```python
from build123d import *

# Parameters (mm, degrees)
F0_R     = 2.9
F1_DEPTH = 15
F1_TAPER = 0.4
F2_DEPTH = 15
F2_TAPER = 0.4
F0_R_2   = 4
F3_DEPTH = 4
F4_DEPTH = 4
F5_R     = 1
F6_R     = 2.1
F7_DEPTH = 4.2
F8_DEPTH = 2.8


with BuildPart() as f1:
    # F0 (on Top) → F1 (new body)
    with BuildSketch(Plane.XY):
        Circle(F0_R)
    extrude(amount=F1_DEPTH, taper=F1_TAPER)

    # F0 (on Top) → F2 (join)
    with BuildSketch(Plane.XY):
        Circle(F0_R)
    extrude(amount=-F2_DEPTH, taper=F2_TAPER)

    # F0 (on Top) → F3 (join)
    with BuildSketch(Plane.XY):
        Circle(F0_R_2)
        Circle(F0_R, mode=Mode.SUBTRACT)
        Circle(F0_R)
    extrude(amount=F3_DEPTH)

    # F0 (on Top) → F4 (join)
    with BuildSketch(Plane.XY):
        Circle(F0_R_2)
        Circle(F0_R, mode=Mode.SUBTRACT)
        Circle(F0_R)
    extrude(amount=-F4_DEPTH)

    # F5
    f5_edges = [f1.edges().sort_by_distance(p)[0] for p in [
        (-2.795279, 0, 15),
        (-2.795279, 0, -15),
    ]]
    fillet(f5_edges, radius=F5_R)

    # F6 (on Front) → F7 (cut)
    with BuildSketch(Plane.XZ):
        Circle(F6_R)
    extrude(amount=-F7_DEPTH, mode=Mode.SUBTRACT)

    # F6 (on Front) → F8 (cut)
    with BuildSketch(Plane.XZ):
        Circle(F6_R)
    extrude(amount=F8_DEPTH, mode=Mode.SUBTRACT)


solid = f1.part
```
The model under review builds one solid part; all positions refer to its coordinate system, in mm. A direction names the side the tool comes from. Coordinates: 2 decimals unless noted, no trailing zeros. Write each loop counter-clockwise with the first axis right and the second up, starting at its lowest first coordinate (ties: lowest second). Pieces come first, ordered by that corner, then holes.
1) We need section A-A on z = -8. State the section outline as (x, y) points.
2) We need section B-B on z = -0.75. State the section outline as (x, y) points.
3) To check wall thickness, follow probe 1 along Z at (x, y) = (0, -1.65); probe 2 along Z at (x, y) = (1, 0.5); probe 3 along X at (y, z) = (-2.25, 0.25). State the ranges of each line that lie inside material, in increasing order.
4) Clearance check with flat-ended pins moving along their axes: pin 1 Ø3.5 at (x, z) = (-0.5, 0) entering from +Y; pin 2 Ø2 at (x, z) = (1, -10) entering from -Y; pin 3 Ø1.5 at (y, z) = (2.5, -1) entering from -X. State where each tip first meets the part, or that it passes through.
5) The part is to be moulded in two halves that separate along X. For faces 4 (the face through (0, 0, -15)), 5 (the face through (-0.61, -2.77, 9.07)), 6 (the face through (0, -2.8, 0)), say which applies: pulls with the +X half, pulls with the -X half, needs draft (parallel to the pull), parting line crosses it, or undercut.
6) Machinability: for faces 1 (the face through (-1, 3, -4)), 2 (the face through (-0.867, -3.905, 0.056)), 3 (the face through (-1, 3, 4)), which of the approach directions +Z, -Z, +X, -X, +Y, -Y give a long, thin tool a straight path to every point of the face, cutting with its end or side? Answer none if there is none.
7) We need section C-C on z = -13. State the section outline as (x, y) points.
Answer list:
1. outline: circle Ø5.69 at (0, 0)
2. outline: (-1.96, -2.8) - (-1.96, 3.49) arc R4 ccw (long way) to (1.96, 3.49) - (1.96, -2.8) - close
3. probe 1: z = -15 to -2.1, 2.1 to 15
3. probe 2: z = -15 to -1.85, 1.85 to 15
3. probe 3: x = -3.31 to -2.09, 2.09 to 3.31
4. pin 1: stops at y = 3.67
4. pin 2: stops at y = -2.83
4. pin 3: stops at x = -3.6
5. face 4: needs draft
5. face 5: parting line crosses it
5. face 6: undercut
6. face 1: -Z
6. face 2: +Z, -Z
6. face 3: +Z
7. outline: circle Ø5.62 at (0, 0)
